Can you work these out from the model? Positions are in its coordinate system, mm. Face numbers are marked on the shaded views. A direction names the side the tool comes from. Coordinates: 2 decimals unless noted, no trailing zeros. Loops run counter-clockwise (first coordinate to the right, second up) from the corner with the lowest first, then second, coordinate; pieces in that order, holes last. Notation, with made-up numbers: (88, 52) -> (116, 52) arc R5 ccw to (116, 61) -> close; hole circle Ø5 at (74.25, -35). An arc over 180 degrees is marked (long way). Put each result on its own line as item: value. Start each with the question number.
Item 1: If we section it at A-A on x = 20.5: Please give me the cut outline in (y, z).
Item 2: If we section it at D-D on z = 12.25: Please give me the cut outline in (x, y), plus the area to 3 significant figures.
Item 3: Please list where these lines run through material, in increasing order: L1, parallel to Z at x = 23, y = 2.95; L2, parallel to Z at x = 0, y = 2.45; L3, parallel to X at y = 1.55, z = 0. Write a range as from..to.
Item 4: If we section it at B-B on z = 0: Please give me the cut outline in (x, y), plus the area to 3 significant figures.
Item 5: We'd pull the mould along X, two halves only. Please class the marked faces 5, 6 and 7: pulls with the +X half, pulls with the -X half, needs draft (parallel to the pull), parting line crosses it, or undercut.
Item 6: If we section it at C-C on y = 2.25: Please give me the cut outline in (x, z).
Item 7: Will these pins go through, and if not, where does the flat tip stop? P1, Ø2, axis at y = 3, z = 2, coming from the -X side; P2, Ø12, axis at x = 10, z = -2.5, coming from the -Y side; P3, Ø1, axis at x = 15.5, y = 1.5, coming from the +Z side; P4, Ø1.5, axis at x = 21, y = 3, coming from the -Z side.
Item 8: For the marked faces 1, 2, 3 and 4, which set-ups out of +Z, -Z, +X, -X, +Y, -Y let a thin tool reach every point of the face, with its end or its side?
```python
from build123d import *

# Parameters (mm, degrees)
BOSS_EXTRUDE1_DEPTH = 5


with BuildPart() as part:
    # Sketch1 → Boss-Extrude1 (new body)
    with BuildSketch(Plane(origin=(0, 0, 0), x_dir=(1, 0, 0), z_dir=(0, 1, 0))):
        with BuildLine():
            Line((4.307841687, -13.95), (31.5, -13.95))
            Line((31.5, -13.95), (31.5, 13.95))
            Line((31.5, 13.95), (4.307841687, 13.95))
            ThreePointArc((4.307841687, 13.95), (-14.6, 0), (4.307841687, -13.95))
        make_face()
        with BuildLine():
            Line((3.472391107, -8.95), (26.5, -8.95))
            Line((26.5, -8.95), (26.5, 8.95))
            Line((26.5, 8.95), (3.472391107, 8.95))
            ThreePointArc((3.472391107, 8.95), (-9.6, 0), (3.472391107, -8.95))
        make_face(mode=Mode.SUBTRACT)
    extrude(amount=BOSS_EXTRUDE1_DEPTH)


solid = part.part
```
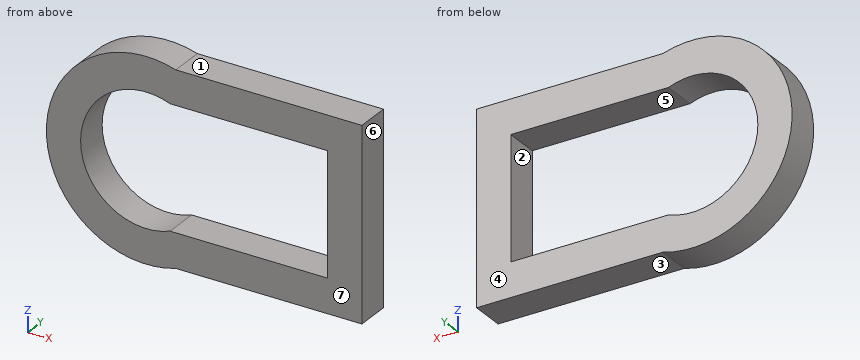
Solutions:
1. outline: (0, -13.95) -> (5, -13.95) -> (5, -8.95) -> (0, -8.95) -> close; (0, 8.95) -> (5, 8.95) -> (5, 13.95) -> (0, 13.95) -> close
2. outline: (-7.94, 0) -> (31.5, 0) -> (31.5, 5) -> (-7.94, 5) -> close
2. area: 197 mm^2
3. L1: -13.95..-8.95, 8.95..13.95
3. L2: -14.6..-9.6, 9.6..14.6
3. L3: -14.6..-9.6, 26.5..31.5
4. outline: (-14.6, 0) -> (-9.6, 0) -> (-9.6, 5) -> (-14.6, 5) -> close; (26.5, 0) -> (31.5, 0) -> (31.5, 5) -> (26.5, 5) -> close
4. area: 50.0 mm^2
5. face 5: undercut
5. face 6: pulls with the +X half
5. face 7: needs draft
6. outline: (4.31, -13.95) -> (31.5, -13.95) -> (31.5, 13.95) -> (4.31, 13.95) arc R14.6 ccw (long way) to start; hole (3.47, -8.95) -> (26.5, -8.95) -> (26.5, 8.95) -> (3.47, 8.95) arc R9.6 ccw (long way) to start
7. P1: x = -14.57
7. P2: through
7. P3: z = 13.95
7. P4: z = -13.95
8. face 1: +Z, +X, +Y, -Y
8. face 2: +Y, -Y
8. face 3: -Z, +X, +Y, -Y
8. face 4: +Z, -Z, +X, -X, +Y
